Can you work these out from the model? Positions are in its coordinate system, mm. A direction names the side the tool comes from. Give positions to 0.01 mm unless a question says otherwise; leave off trailing zeros. Answer as a JSON object with one key per item and string values.
```python
from build123d import *

# Parameters (mm, degrees)
BOSS_EXTRUDE1_DEPTH     = 38.1
SKETCH2_R               = 10.8585
CUT_EXTRUDE1_DEPTH      = 25.4
SKETCH3_R               = 10.8585
CUT_EXTRUDE2_DEPTH      = 25.4
FILLET1_R               = 10
SKETCH5_W               = 26.289
SKETCH5_H               = 26.289
BOSS_EXTRUDE2_DEPTH     = 8.89
SKETCH6_R               = 8.0645
CUT_EXTRUDE3_DEPTH      = 6.35
SKETCH7_R               = 6.35
CUT_EXTRUDE4_DEPTH      = 5.08
FILLET3_R               = 12.7
FILLET4_R               = 5.08
FILLET5_R               = 12.7
CUT_EXTRUDE5_DEPTH      = 191.631332173
CUT_EXTRUDE5_DEPTH_BACK = 191.631332173
SKETCH8_R               = 1.349999967
CUT_EXTRUDE6_DEPTH      = 191.631332193
CUT_EXTRUDE6_DEPTH_BACK = 191.631332193
FILLET6_R               = 2.54


with BuildPart() as part:
    # Sketch1 → Boss-Extrude1 (new body)
    with BuildSketch(Plane(origin=(0, 0, 0), x_dir=(1, 0, 0), z_dir=(0, 1, 0))):
        Polygon((-15.781536726, 38.1), (0, 38.1), (20.791856291, 25.4), (121.448143709, 25.4), (142.24, 38.1), (158.021536726, 38.1), (184.96230509, 11.159231637), (158.021536726, -15.781536726), (142.24, 0), (0, 0), (-15.781536726, -15.781536726), (-42.72230509, 11.159231637), align=None)
    extrude(amount=BOSS_EXTRUDE1_DEPTH)

    # Sketch2 → Cut-Extrude1 (cut)
    with BuildSketch(Plane(origin=(-15.781536726, 0, 15.781536726), x_dir=(0.7071067811865477, 0, 0.7071067811865475), z_dir=(-0.7071067811865475, 0, 0.7071067811865477))):
        with Locations((-19.05, 19.05)):
            Circle(SKETCH2_R)
    extrude(amount=-CUT_EXTRUDE1_DEPTH, mode=Mode.SUBTRACT)

    # Sketch3 → Cut-Extrude2 (cut)
    with BuildSketch(Plane(origin=(86.901536726, 0, 86.901536726), x_dir=(0.7071067811865478, 0, -0.7071067811865474), z_dir=(0.7071067811865474, 0, 0.7071067811865478))):
        with Locations((119.628868556, 19.05)):
            Circle(SKETCH3_R)
    extrude(amount=-CUT_EXTRUDE2_DEPTH, mode=Mode.SUBTRACT)

    # Fillet1
    fillet1_edges = [part.edges().sort_by_distance(p)[0] for p in [
        (142.24, 19.05, 0),
        (0, 19.05, 0),
    ]]
    fillet(fillet1_edges, radius=FILLET1_R)

    # Sketch5 → Boss-Extrude2 (add)
    with BuildSketch(Plane.XY):
        with Locations((71.12, 13.1445)):
            Rectangle(SKETCH5_W, SKETCH5_H)
    extrude(amount=BOSS_EXTRUDE2_DEPTH)

    # Sketch6 → Cut-Extrude3 (cut)
    with BuildSketch(Plane.XY.offset(8.89)):
        with Locations((71.12, 13.1445)):
            Circle(SKETCH6_R)
    extrude(amount=-CUT_EXTRUDE3_DEPTH, mode=Mode.SUBTRACT)

    # Sketch7 → Cut-Extrude4 (cut)
    with BuildSketch(Plane.XY.offset(2.54)):
        with Locations((71.12, 13.1445)):
            Circle(SKETCH7_R)
    extrude(amount=-CUT_EXTRUDE4_DEPTH, mode=Mode.SUBTRACT)

    # Fillet3
    fillet3_edges = [part.edges().sort_by_distance(p)[0] for p in [
        (57.9755, 26.289, 4.445),
        (84.2645, 26.289, 4.445),
    ]]
    fillet(fillet3_edges, radius=FILLET3_R)

    # Fillet4
    fillet4_edges = [part.edges().sort_by_distance(p)[0] for p in [
        (-29.251920908, 0, 2.311152545),
        (171.491920908, 0, 2.311152545),
        (171.491920908, 38.1, 2.311152545),
        (-15.781536726, 19.05, 15.781536726),
        (-42.72230509, 19.05, -11.159231637),
        (184.96230509, 19.05, -11.159231637),
        (158.021536726, 19.05, 15.781536726),
        (-29.251920908, 38.1, 2.311152545),
    ]]
    fillet(fillet4_edges, radius=FILLET4_R)

    # Fillet5
    fillet5_edges = [part.edges().sort_by_distance(p)[0] for p in [
        (-15.781536726, 19.05, -38.1),
        (0, 19.05, -38.1),
        (20.791856291, 19.05, -25.4),
        (121.448143709, 19.05, -25.4),
        (142.24, 19.05, -38.1),
        (158.021536726, 19.05, -38.1),
    ]]
    fillet(fillet5_edges, radius=FILLET5_R)

    # Sketch8 → Cut-Extrude5 (cut, two sides: drawn at the far end of the back side and taken through both)
    with BuildSketch(Plane(origin=(0, 38.1, 0), x_dir=(1, 0, 0), z_dir=(0, 1, 0)).offset(-CUT_EXTRUDE5_DEPTH_BACK)):
        with Locations(Location((-20.271664787, 6.669103576, 0), (0, 0, 270))):
            Circle(SKETCH8_R)
        with Locations(Location((162.511664787, 6.669103576, 0), (0, 0, 270))):
            Circle(SKETCH8_R)
    extrude(amount=CUT_EXTRUDE5_DEPTH + CUT_EXTRUDE5_DEPTH_BACK, mode=Mode.SUBTRACT)

    # Sketch9 → Cut-Extrude6 (cut, two sides: drawn at the far end of the back side and taken through both)
    with BuildSketch(Plane.XY.offset(-CUT_EXTRUDE6_DEPTH_BACK)):
        Polygon((12.7, 9.525), (38.1, 9.525), (57.15, 28.575), (31.75, 28.575), align=None)
        Polygon((85.09, 28.575), (110.49, 28.575), (129.54, 9.525), (104.14, 9.525), align=None)
    extrude(amount=CUT_EXTRUDE6_DEPTH + CUT_EXTRUDE6_DEPTH_BACK, mode=Mode.SUBTRACT)

    # Fillet6
    fillet6_edges = [part.edges().sort_by_distance(p)[0] for p in [
        (129.54, 9.525, -15.17131794),
        (110.49, 28.575, -12.7),
        (85.09, 28.575, -12.7),
        (104.14, 9.525, -12.7),
        (38.1, 9.525, -12.7),
        (57.15, 28.575, -12.7),
        (31.75, 28.575, -12.7),
        (12.7, 9.525, -15.17131794),
    ]]
    fillet(fillet6_edges, radius=FILLET6_R)


solid = part.part
```
1. If we mould it in two halves opening along Z, with no side actions, what happens to faces 1 (the face through (100, 28.575, -13)), 2 (the face through (20.97, 4.95, -25.86)), 3 (the face through (166.765, 28.206, -10.671)), 4 (the face through (72, 27, 0))? For each: +Z half, -Z half, draft (parallel to the pull), parting line (faces both ways), or undercut.
Worked answers:
{"face 1": "draft", "face 2": "-Z half", "face 3": "undercut", "face 4": "+Z half"}
2. For faces 5 (the face through (57.976, 7, 4)), 6 (the face through (88.892, 27.046, -12.522)), 7 (the face through (61.597, 22.47, 4.507)), which set-ups out of +Z, -Z, +X, -X, +Y, -Y let a thin tool reach every point of the face, with its end or its side?
Worked answers:
{"face 5": "+Z, +Y, -Y", "face 6": "+Z, -Z", "face 7": "+Z, +Y"}
3. Will these pins go through, and if not, where does the flat tip stop? pin 1 Ø10 at (y, z) = (7.5, -20.5) entering from -X; pin 2 Ø2.5 at (x, z) = (-20.27, -6.67) entering from -Y; pin 3 Ø19 at (x, y) = (88, 27.5) entering from -Z; pin 4 Ø2 at (y, z) = (25, 7) entering from +X.
Worked answers:
{"pin 1": "x = -38.38", "pin 2": "through", "pin 3": "z = -25.4", "pin 4": "x = 164.76"}
4. Please list where these lines run through material, in increasing order: L1, parallel to X at y = 20, z = -1.5 (3 decimals); L2, parallel to X at y = 18.5, z = -4 (3 decimals); L3, parallel to X at y = 10, z = 8.5.
Worked answers:
{"L1": "-10.143 to 23.175, 48.575 to 93.665, 119.065 to 152.383", "L2": "-7.604 to 21.675, 47.075 to 95.165, 120.565 to 149.844", "L3": "-23.06 to -8.5, 57.98 to 63.69, 78.55 to 84.26, 150.74 to 165.3"}
